```python
from build123d import *

# Parameters (mm, degrees)
SKETCH_1_R      = 2.5
EXTRUDE_1_DEPTH = 8


with BuildPart() as part:
    # 草图1 → 凸台-拉伸1 (new body)
    with BuildSketch(Plane.XY):
        with BuildLine():
            Line((-100.826455741, 4.931224078), (47.520632777, 29.793672234))
            ThreePointArc((47.520632777, 29.793672234), (52.376150378, 29.81060125), (56.982686096, 28.27562032))
            Line((56.982686096, 28.27562032), (102.327562032, 4.425206773))
            ThreePointArc((102.327562032, 4.425206773), (105, 0), (102.327562032, -4.425206773))
            Line((102.327562032, -4.425206773), (56.982686096, -28.27562032))
            ThreePointArc((56.982686096, -28.27562032), (52.376150378, -29.81060125), (47.520632777, -29.793672234))
            Line((47.520632777, -29.793672234), (-100.826455741, -4.931224078))
            ThreePointArc((-100.826455741, -4.931224078), (-105, 0), (-100.826455741, 4.931224078))
        make_face()
        with Locations((85, 0)):
            Circle(SKETCH_1_R, mode=Mode.SUBTRACT)
        with Locations((67.679491924, 10)):
            Circle(SKETCH_1_R, mode=Mode.SUBTRACT)
        with Locations(Location((67.679491924, -10, 0), (0, 0, 180))):
            Circle(SKETCH_1_R, mode=Mode.SUBTRACT)
        with Locations((-90, 0)):
            Circle(SKETCH_1_R, mode=Mode.SUBTRACT)
    extrude(amount=EXTRUDE_1_DEPTH)


solid = part.part
```
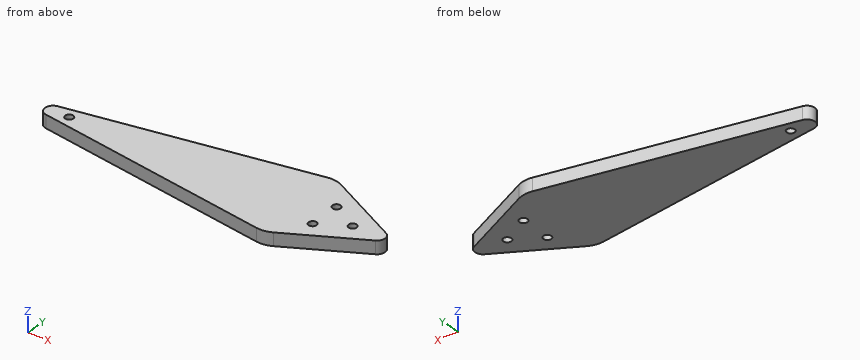
The listing builds one solid part. Answer for the finished solid, in the listing's coordinates (mm). Coordinates: 2 decimals unless noted, no trailing zeros. Loops run counter-clockwise (first coordinate to the right, second up) from the corner with the lowest first, then second, coordinate; pieces in that order, holes last. Notation, with made-up numbers: (29, 68.25) - (63, 68.25) arc R29 ccw to (63, 93.25) - close; hole circle Ø3 at (-17, 59). An arc over 180 degrees is marked (long way). Use a Markdown table: item, result. Add a question column.
1) The part is cut by section D-D, the plane y = -10. Give the vertices of the cut face in (x, z).
2) The part is cut by section C-C, the plane y = 0. Give the vertices of the cut face in (x, z), and give its area (3 significant figures).
3) The part is cut by section A-A, the plane z = 3.25. Give the vertices of the cut face in (x, y).
4) The part is cut by section B-B, the plane x = 85. Give the vertices of the cut face in (y, z), and give its area (3 significant figures).
5) Find the intervals of material crossed by line 1 (Y direction, x = 32, z = 4.75); line 2 (Y direction, x = -60, z = 5.75), in increasing order.
6) Given pin 1 (2 mm diameter, centred on y = -10.5, z = 6, fed in from +X); pin 2 (1.5 mm diameter, centred on x = -43, z = 2, fed in from +Y); pin 3 (1 mm diameter, centred on x = 68.5, z = 2.5, fed in from +Y); pin 4 (3 mm diameter, centred on x = -90, y = 0, fed in from -Z), each flat-ended and moving along its own axis, determine where each tip first touches the part or whether it passes through.
Here are the results:
| question | item | result |
|---|---|---|
| 1 | outline | (-70.58, 0) - (65.18, 0) - (65.18, 8) - (-70.58, 8) - close; (70.18, 0) - (91.73, 0) - (91.73, 8) - (70.18, 8) - close |
| 2 | outline | (-105, 0) - (-92.5, 0) - (-92.5, 8) - (-105, 8) - close; (-87.5, 0) - (82.5, 0) - (82.5, 8) - (-87.5, 8) - close; (87.5, 0) - (105, 0) - (105, 8) - (87.5, 8) - close |
| 2 | area | 1,600 mm^2 |
| 3 | outline | (-100.83, -4.93) - (47.52, -29.79) arc R15 ccw to (56.98, -28.28) - (102.33, -4.43) arc R5 ccw to (102.33, 4.43) - (56.98, 28.28) arc R15 ccw to (47.52, 29.79) - (-100.83, 4.93) arc R5 ccw to start; hole circle Ø5 at (-90, 0); hole circle Ø5 at (67.68, -10); hole circle Ø5 at (67.68, 10); hole circle Ø5 at (85, 0) |
| 4 | outline | (-13.54, 0) - (-2.5, 0) - (-2.5, 8) - (-13.54, 8) - close; (2.5, 0) - (13.54, 0) - (13.54, 8) - (2.5, 8) - close |
| 4 | area | 177 mm^2 |
| 5 | line 1 | y = -27.19 to 27.19 |
| 5 | line 2 | y = -11.77 to 11.77 |
| 6 | pin 1 | stops at x = 92.68 |
| 6 | pin 2 | stops at y = 14.75 |
| 6 | pin 3 | stops at y = 22.48 |
| 6 | pin 4 | passes through |
